The listing builds one solid part. Answer for the finished solid, in the listing's coordinates (mm). A direction names the side the tool comes from. Give positions to 0.01 mm unless a question says otherwise; leave off trailing zeros. Write each loop counter-clockwise with the first axis right and the second up, starting at its lowest first coordinate (ties: lowest second). Pieces come first, ordered by that corner, then holes. Notation, with made-up numbers: (37, -22.75) - (83, -22.75) arc R15 cw to (83, 0.25) - close; hole circle Ø4 at (19.25, 63). An arc over 180 degrees is marked (long way). Answer as CSV lines item,"result". Start each with the question number.
(1) Find section D-D (y = 4). Write down the section's boundary in (x, z) (3 decimals), then the cut area to 3 significant figures.
(2) Find section C-C (z = -5). Write down the section's boundary in (x, y) (3 decimals).
(3) Each of these flat-tipped pins is pushed along its axis until it touches: pin 1 Ø10.5 at (y, z) = (-13, -8.5) entering from +X (3 decimals); pin 2 Ø6 at (x, y) = (12, -17.5) entering from -Z; pin 3 Ø5 at (y, z) = (2, -14) entering from -X. Where does it stop, or does it pass through?
(4) For faces 1 (the face through (5, 0, -13)), 2 (the face through (0, -13, -10)), 3 (the face through (9.525, -13, -11)), determine the directions among +Z, -Z, +X, -X, +Y, -Y from which every point of the face is accessible in a straight line to the end or side of a thin tool.
(5) Straight lines are drawn through the part: probe 1 along Y at (x, z) = (1.75, -8); probe 2 along Z at (x, y) = (-7.5, 0.5); probe 3 along X at (y, z) = (-15.5, -6.5) (3 decimals). For each, find the intervals that lie inside material, in ascending order.
(6) Find section B-B (x = 7.75). Write down the section's boundary in (y, z) (3 decimals).
from build123d import *

# Parameters (mm, degrees)
F1_DEPTH = 25.4
F3_DEPTH = 34.925
F4_W     = 28.575
F4_H     = 6.45089
F5_DEPTH = 9.525


with BuildPart() as f1:
    # F0 (on Front) → F1 (new body)
    with BuildSketch(Plane.XZ):
        Polygon((9.525, 0), (0, 0), (0, -20.954376), (4.7625, -25.4), (9.525, -20.954376), align=None)
    extrude(amount=F1_DEPTH)

    # F2 (on face) → F3 (join)
    with BuildSketch(Plane(origin=(0, 0, 0), x_dir=(-1, 0, 0), z_dir=(0, 1, 0))):
        Polygon((-19.05, 6.45089), (-19.05, 0), (-9.525, 0), (0, 0), (9.525, 0), (9.525, 6.45089), align=None)
    extrude(amount=-F3_DEPTH)

    # F4 (on face) → F5 (join)
    with BuildSketch(Plane(origin=(0, 0, 0), x_dir=(-1, 0, 0), z_dir=(0, 1, 0))):
        with Locations((-4.7625, 3.225445)):
            Rectangle(F4_W, F4_H)
    extrude(amount=F5_DEPTH)


solid = f1.part
Result set:
1,outline,"(-9.525, 0) - (19.05, 0) - (19.05, 6.451) - (-9.525, 6.451) - close"
1,area,"184 mm^2"
2,outline,"(0, -25.4) - (9.525, -25.4) - (9.525, 0) - (0, 0) - close"
3,pin 1,"x = 9.525"
3,pin 2,"z = -21.44"
3,pin 3,"x = 0"
4,face 1,"-Z, +X, -X, +Y"
4,face 2,"-Z, -X, +Y, -Y"
4,face 3,"-Z, +X, +Y, -Y"
5,probe 1,"-25.4 to 0"
5,probe 2,"0 to 6.45"
5,probe 3,"0 to 9.525"
6,outline,"(-34.925, 0) - (-25.4, 0) - (-25.4, -22.611) - (0, -22.611) - (0, 0) - (9.525, 0) - (9.525, 6.451) - (-34.925, 6.451) - close"
